Part model, mm, in its own coordinate system. A direction names the side the tool comes from. Round coordinates to 2 decimals unless told otherwise and drop trailing zeros. Loops run counter-clockwise (first coordinate to the right, second up) from the corner with the lowest first, then second, coordinate; pieces in that order, holes last.
from build123d import *

# Parameters (mm, degrees)
BOSS_EXTRUDE1_DEPTH = 25
SKETCH2_W           = 101
SKETCH2_H           = 39
BOSS_EXTRUDE2_DEPTH = 2
CUT_EXTRUDE1_DEPTH  = 1


with BuildPart() as part:
    # Sketch1 → Boss-Extrude1 (new body)
    with BuildSketch(Plane(origin=(0, 0, 0), x_dir=(1, 0, 0), z_dir=(0, 1, 0))):
        Polygon((0, 39), (0, 32), (2, 32), (2, 37), (99, 37), (99, 2), (2, 2), (2, 17), (0, 17), (0, 0), (101, 0), (101, 39), align=None)
    extrude(amount=BOSS_EXTRUDE1_DEPTH)

    # Sketch2 → Boss-Extrude2 (add)
    with BuildSketch(Plane(origin=(0, 0, 0), x_dir=(-1, 0, 0), z_dir=(0, -1, 0))):
        with Locations((-50.5, 19.5)):
            Rectangle(SKETCH2_W, SKETCH2_H)
    extrude(amount=BOSS_EXTRUDE2_DEPTH)

    # Sketch3 → Cut-Extrude1 (cut)
    with BuildSketch(Plane(origin=(0, 25, 0), x_dir=(1, 0, 0), z_dir=(0, 1, 0))):
        Polygon((2, 32), (1, 32), (1, 38), (100, 38), (100, 1), (1, 1), (1, 17), (2, 17), (2, 2), (99, 2), (99, 37), (2, 37), align=None)
    extrude(amount=-CUT_EXTRUDE1_DEPTH, mode=Mode.SUBTRACT)


solid = part.part
1) Tool access for faces 4 (the face through (2, 12, -9)), 5 (the face through (1, 12, -17)), 6 (the face through (51, 12, -39)): list every direction of +Z, -Z, +X, -X, +Y, -Y with a clear straight run to the whole face (end or side of a thin tool).
Values:
face 4: +Y
face 5: -X, +Y
face 6: -Z, +X, -X, +Y, -Y
2) Wall check: line 1 along Z through (x, y) = (24.5, 21.5); line 2 along X through (y, z) = (8.75, -9.5); line 3 along Y through (x, z) = (44.5, -6). Give the ranges that are in metal, low to high.
Values:
line 1: z = -39 to -37, -2 to 0
line 2: x = 0 to 2, 99 to 101
line 3: y = -2 to 0
3) Drop a flat-ended pin along its axis: pin 1 Ø6 at (x, z) = (76.5, -31.5) entering from +Y. Give the stop position or say it passes through.
Values:
pin 1: stops at y = 0
4) Slice it at A-A, the plane z = -30. Give the cut face in (x, y), then the cut area to 3 significant figures.
Values:
outline: (0, -2) - (101, -2) - (101, 25) - (100, 25) - (100, 24) - (99, 24) - (99, 0) - (0, 0) - close
area: 251 mm2
5) Slice it at C-C, the plane y = 3.5. Give the cut face in (x, z), then the cut area to 3 significant figures.
Values:
outline: (0, -39) - (101, -39) - (101, 0) - (0, 0) - (0, -17) - (2, -17) - (2, -2) - (99, -2) - (99, -37) - (2, -37) - (2, -32) - (0, -32) - close
area: 514 mm2
6) Mould opens along X. For faces 1 (the face through (0, 12, -15)), 2 (the face through (1, 12, -32)), 3 (the face through (50, 0, -20)) say: released by +X, released by -X, zero draft, split by the parting line, or undercut.
Values:
face 1: released by -X
face 2: zero draft
face 3: undercut
7) Slice it at B-B, the plane x = 47. Give the cut face in (y, z), then the cut area to 3 significant figures.
Values:
outline: (-2, -39) - (25, -39) - (25, -38) - (24, -38) - (24, -37) - (0, -37) - (0, -2) - (24, -2) - (24, -1) - (25, -1) - (25, 0) - (-2, 0) - close
area: 176 mm2
